Job drawing, mm, ordinate dimensions from the low corner. One solid piece. A direction names the side the tool comes from. Give positions to 0.01 mm unless a question says otherwise; leave off trailing zeros. Order: outer loops, then holes, each group sorted by start corner. A loop starts at its lowest first (then second) coordinate and runs counter-clockwise, first axis right, second up.
1. Slice it at C-C on z = 61. List the corners of the cut face in (x, y).
2. Slice it at B-B on y = 17. List the corners of the cut face in (x, z).
3. Drop flat-ended pins along their axis: pin 1 Ø3.5 at (x, z) = (135.89, 3.81) entering from +Y; pin 2 Ø10 at (x, z) = (104, 44.5) entering from +Y. Give the stop position or say it passes through.
4. Slice it at D-D on x = 3.81. List the corners of the cut face in (y, z) (1 decimal), and give its area (3 significant figures).
5. Which spindle directions (+Z, -Z, +X, -X, +Y, -Y) get a long thin tool onto all of the face, cutting with end or side? Do the marked faces 1 and 2. Say none if no direction does.
6. Mould opens along Z. For the marked faces 3, 4 and 5 say: +Z half, -Z half, draft (parallel to the pull), parting line (faces both ways), or undercut.
7. Probe line 1 (X direction, y = 42.5, z = 85.09) (1 decimal); line 2 (Z direction, x = 91.5, y = 24); line 3 (X direction, y = 14.5, z = 13.5). List the from-to ranges inside material, lowest first.
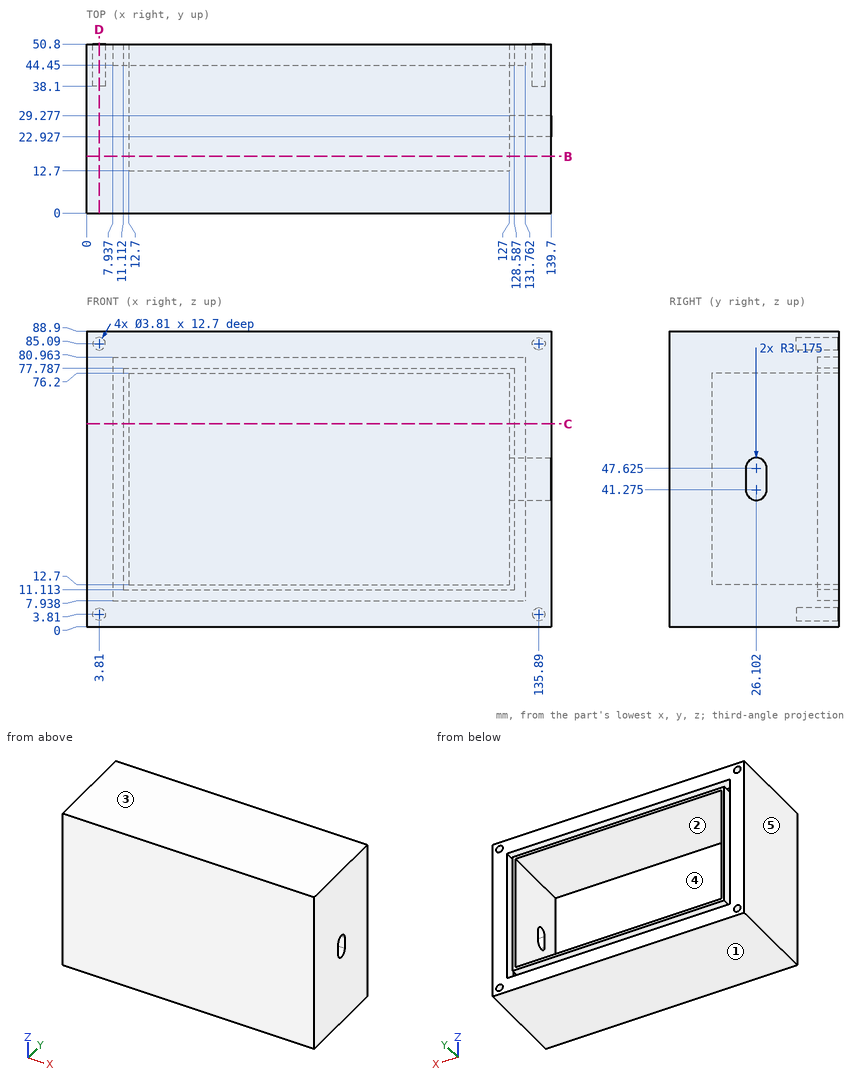
Data:
1. outline: (0, 0) - (139.7, 0) - (139.7, 50.8) - (131.76, 50.8) - (131.76, 44.45) - (128.59, 44.45) - (128.59, 50.8) - (127, 50.8) - (127, 12.7) - (12.7, 12.7) - (12.7, 50.8) - (11.11, 50.8) - (11.11, 44.45) - (7.94, 44.45) - (7.94, 50.8) - (0, 50.8) - close
2. outline: (0, 0) - (139.7, 0) - (139.7, 88.9) - (0, 88.9) - close; hole (12.7, 12.7) - (127, 12.7) - (127, 76.2) - (12.7, 76.2) - close
3. pin 1: stops at y = 38.1
3. pin 2: stops at y = 12.7
4. outline: (0, 0) - (50.8, 0) - (50.8, 1.9) - (38.1, 1.9) - (38.1, 5.7) - (50.8, 5.7) - (50.8, 83.2) - (38.1, 83.2) - (38.1, 87) - (50.8, 87) - (50.8, 88.9) - (0, 88.9) - close
4. area: 4,420 mm2
5. face 1: -Z, +X, -X, +Y, -Y
5. face 2: +Y
6. face 3: +Z half
6. face 4: undercut
6. face 5: draft
7. line 1: x = 0 to 1.9, 5.7 to 134, 137.8 to 139.7
7. line 2: z = 0 to 12.7, 76.2 to 88.9
7. line 3: x = 0 to 12.7, 127 to 139.7
